```python
from build123d import *

# Parameters (mm, degrees)
SKETCH1_R               = 72.5
SKETCH1_R_2             = 62.5
BOSS_EXTRUDE1_DEPTH     = 10
SKETCH2_W               = 25
SKETCH2_H               = 10
BOSS_EXTRUDE2_DEPTH     = 100
SKETCH3_W               = 145
SKETCH3_H               = 50
BOSS_EXTRUDE3_DEPTH     = 10
CUT_EXTRUDE1_START      = -10
SKETCH4_R               = 62.5
CUT_EXTRUDE1_DEPTH      = 10
SKETCH5_W               = 145
SKETCH5_H               = 12.5
BOSS_EXTRUDE4_DEPTH     = 50
CUT_EXTRUDE2_DEPTH      = 138.318061449
CUT_EXTRUDE2_DEPTH_BACK = 138.318061449
SKETCH6_R               = 3.5
CUT_EXTRUDE3_DEPTH      = 138.318061449
CUT_EXTRUDE3_DEPTH_BACK = 138.318061449
SKETCH7_W               = 3.75
SKETCH7_H               = 5


with BuildPart() as part:
    # Sketch1 → Boss-Extrude1 (new body)
    with BuildSketch(Plane(origin=(0, 0, 0), x_dir=(1, 0, 0), z_dir=(0, 1, 0))):
        with Locations(Location((0, 0, 0), (0, 0, 270))):
            Circle(SKETCH1_R)
        with Locations(Location((0, 0, 0), (0, 0, 270))):
            Circle(SKETCH1_R_2, mode=Mode.SUBTRACT)
    extrude(amount=BOSS_EXTRUDE1_DEPTH)

    # Sketch2 → Boss-Extrude2 (add)
    with BuildSketch(Plane.XY):
        with Locations((-60, 5)):
            Rectangle(SKETCH2_W, SKETCH2_H)
        with Locations((60, 5)):
            Rectangle(SKETCH2_W, SKETCH2_H)
    extrude(amount=BOSS_EXTRUDE2_DEPTH)

    # Sketch3 → Boss-Extrude3 (add)
    with BuildSketch(Plane(origin=(0, 10, 0), x_dir=(1, 0, 0), z_dir=(0, 1, 0))):
        with Locations((0, -75)):
            Rectangle(SKETCH3_W, SKETCH3_H)
    extrude(amount=-BOSS_EXTRUDE3_DEPTH)

    # Sketch4 → Cut-Extrude1 (cut)
    with BuildSketch(Plane(origin=(0, 10, 0), x_dir=(1, 0, 0), z_dir=(0, 1, 0)).offset(CUT_EXTRUDE1_START)):
        with Locations(Location((0, 0, 0), (0, 0, 270))):
            Circle(SKETCH4_R)
    extrude(amount=CUT_EXTRUDE1_DEPTH, mode=Mode.SUBTRACT)

    # Sketch5 → Boss-Extrude4 (add)
    with BuildSketch(Plane(origin=(0, 10, 0), x_dir=(1, 0, 0), z_dir=(0, 1, 0))):
        with Locations((0, -93.75)):
            Rectangle(SKETCH5_W, SKETCH5_H)
    extrude(amount=BOSS_EXTRUDE4_DEPTH)

    # Sketch6 → Cut-Extrude2 (cut, two sides: drawn at the far end of the back side and taken through both)
    with BuildSketch(Plane.XZ.offset(-CUT_EXTRUDE2_DEPTH_BACK)):
        with Locations(Location((-50.65, 95, 0), (0, 0, 270))):
            Circle(SKETCH6_R)
        with Locations(Location((-16.9, 95, 0), (0, 0, 270))):
            Circle(SKETCH6_R)
        with Locations(Location((16.85, 95, 0), (0, 0, 270))):
            Circle(SKETCH6_R)
        with Locations(Location((50.6, 95, 0), (0, 0, 270))):
            Circle(SKETCH6_R)
    extrude(amount=CUT_EXTRUDE2_DEPTH + CUT_EXTRUDE2_DEPTH_BACK, mode=Mode.SUBTRACT)

    # Sketch7 → Cut-Extrude3 (cut, two sides: drawn at the far end of the back side and taken through both)
    with BuildSketch(Plane.XZ.offset(-CUT_EXTRUDE3_DEPTH_BACK)):
        with Locations((-16.9, 100)):
            Rectangle(SKETCH7_W, SKETCH7_H)
        with Locations((-50.65, 100)):
            Rectangle(SKETCH7_W, SKETCH7_H)
        with Locations((16.85, 100)):
            Rectangle(SKETCH7_W, SKETCH7_H)
        with Locations((50.6, 100)):
            Rectangle(SKETCH7_W, SKETCH7_H)
    extrude(amount=CUT_EXTRUDE3_DEPTH + CUT_EXTRUDE3_DEPTH_BACK, mode=Mode.SUBTRACT)


solid = part.part
```
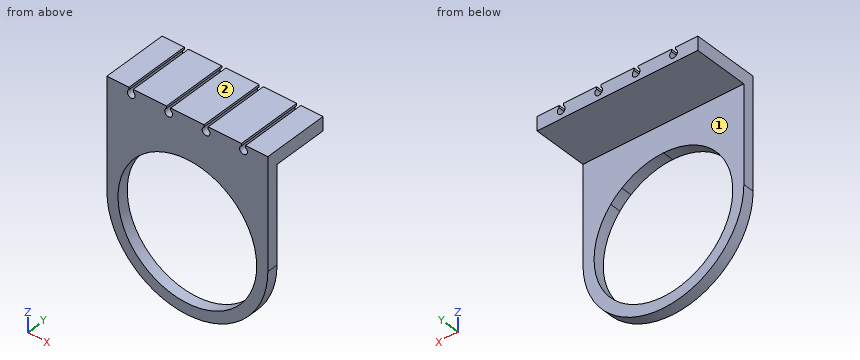
The listing builds one solid part. Answer for the finished solid, in the listing's coordinates (mm). Face numbers are marked on the shaded views. A direction names the side the tool comes from. Round coordinates to 2 decimals unless told otherwise and drop trailing zeros. Order: outer loops, then holes, each group sorted by start corner. A loop starts at its lowest first (then second) coordinate and runs counter-clockwise, first axis right, second up. Notation, with made-up numbers: (11.5, 9) -> (17.5, 9) arc R32 ccw to (17.5, 42) -> close; hole circle Ø6 at (53.5, -10.5). An arc over 180 degrees is marked (long way). Answer as CSV lines item,"result".
Q1. A cutting plane is placed at D-D on z = -35. Determine the outline of the cut face in (x, y), plus the area to 3 significant figures.
Computed values:
outline,"(-63.49, 0) -> (-51.78, 0) -> (-51.78, 10) -> (-63.49, 10) -> close; (51.78, 0) -> (63.49, 0) -> (63.49, 10) -> (51.78, 10) -> close"
area,"234 mm^2"
Q2. A cutting plane is placed at A-A on z = 95. Determine the outline of the cut face in (x, y), plus the area to 3 significant figures.
Computed values:
outline,"(-72.5, 0) -> (-54.15, 0) -> (-54.15, 60) -> (-72.5, 60) -> close; (-47.15, 0) -> (-20.4, 0) -> (-20.4, 60) -> (-47.15, 60) -> close; (-13.4, 0) -> (13.35, 0) -> (13.35, 60) -> (-13.4, 60) -> close; (20.35, 0) -> (47.1, 0) -> (47.1, 60) -> (20.35, 60) -> close; (54.1, 0) -> (72.5, 0) -> (72.5, 60) -> (54.1, 60) -> close"
area,"7,020 mm^2"
Q3. A cutting plane is placed at B-B on x = 32.5. Determine the outline of the cut face in (y, z), plus the area to 3 significant figures.
Computed values:
outline,"(0, -64.81) -> (10, -64.81) -> (10, -53.39) -> (0, -53.39) -> close; (0, 53.39) -> (10, 53.39) -> (10, 87.5) -> (60, 87.5) -> (60, 100) -> (0, 100) -> close"
area,"1,210 mm^2"
Q4. Given pin 1 (5.5 mm diameter, centred on x = -50.65, z = 95, fed in from -Y), flat-ended and moving along its own axis, determine where the tip first touches the part or whether it passes through.
Computed values:
pin 1,"passes through"
Q5. Consider line 1 (X direction, y = 20, z = 95); line 2 (Y direction, x = -3, z = 77); line 3 (Z direction, x = -45.5, y = 47.5). Determine where each line is inside the solid, lowest interval first. Write a range as from..to.
Computed values:
line 1,"x = -72.5..-54.15, -47.15..-20.4, -13.4..13.35, 20.35..47.1, 54.1..72.5"
line 2,"y = 0..10"
line 3,"z = 87.5..100"
Q6. Which of the six approach directions +Z, -Z, +X, -X, +Y, -Y give full straight-line access (tool end or side, diameter ignored) to the marked faces 1 and 2?
Computed values:
face 1,"-Z, +X, -X, +Y"
face 2,"+Z, +X, -X, +Y, -Y"
Q7. A cutting plane is placed at C-C on y = 25. Determine the outline of the cut face in (x, z) (3 decimals), plus the area to 3 significant figures.
Computed values:
outline,"(-72.5, 87.5) -> (72.5, 87.5) -> (72.5, 100) -> (52.475, 100) -> (52.475, 97.955) arc R3.5 cw (long way) to (48.725, 97.955) -> (48.725, 100) -> (18.725, 100) -> (18.725, 97.955) arc R3.5 cw (long way) to (14.975, 97.955) -> (14.975, 100) -> (-15.025, 100) -> (-15.025, 97.955) arc R3.5 cw (long way) to (-18.775, 97.955) -> (-18.775, 100) -> (-48.775, 100) -> (-48.775, 97.955) arc R3.5 cw (long way) to (-52.525, 97.955) -> (-52.525, 100) -> (-72.5, 100) -> close"
area,"1,630 mm^2"
